Design review of the part shown in the three views and the two pictorial views. Dimensions are in mm from the part's minimum x, y and z. Give positions to 0.01 mm unless a question says otherwise; leave off trailing zeros. Write each loop counter-clockwise with the first axis right and the second up, starting at its lowest first coordinate (ties: lowest second). Pieces come first, ordered by that corner, then holes. Notation, with made-up numbers: M 14,18 L 56,18 A10 cw 56,34 Z; hole C 4.5,-7.75 d7. An arc over 180 degrees is marked long. Use one line per item in the form item = value. Start each with the question number.
Q1. Consider section D-D on z = 14. Write out the cut boundary in (x, y) (3 decimals).
Q2. For probe 1 along X at (y, z) = (2.5, 16.05) (3 decimals); probe 2 along Y at (x, z) = (1.1, 15.5) (1 decimal); probe 3 along Y at (x, z) = (1.05, 2.5) (1 decimal), list the stretches that pass through material, from the lowest coordinate up. Write a range as [from, to].
Q3. Clearance check with flat-ended pins moving along their axes: pin 1 Ø2 at (x, z) = (3.5, 3.5) entering from -Y; pin 2 Ø1 at (x, z) = (2.5, 12) entering from -Y; pin 3 Ø2 at (x, y) = (2.17, 2.5) entering from +Z. State where each tip first meets the part, or that it passes through.
Q4. Consider section C-C on x = 0.4. Write out the cut boundary in (y, z), and give its area (3 significant figures).
Q5. Mouldability with a two-part tool opening along Y and no side actions: class the marked faces 1, 2, 3 and 4 as released by +Y, released by -Y, zero draft, split by the parting line, or undercut.
Q6. Consider section A-A on z = 2.75. Write out the cut boundary in (x, y) (3 decimals).
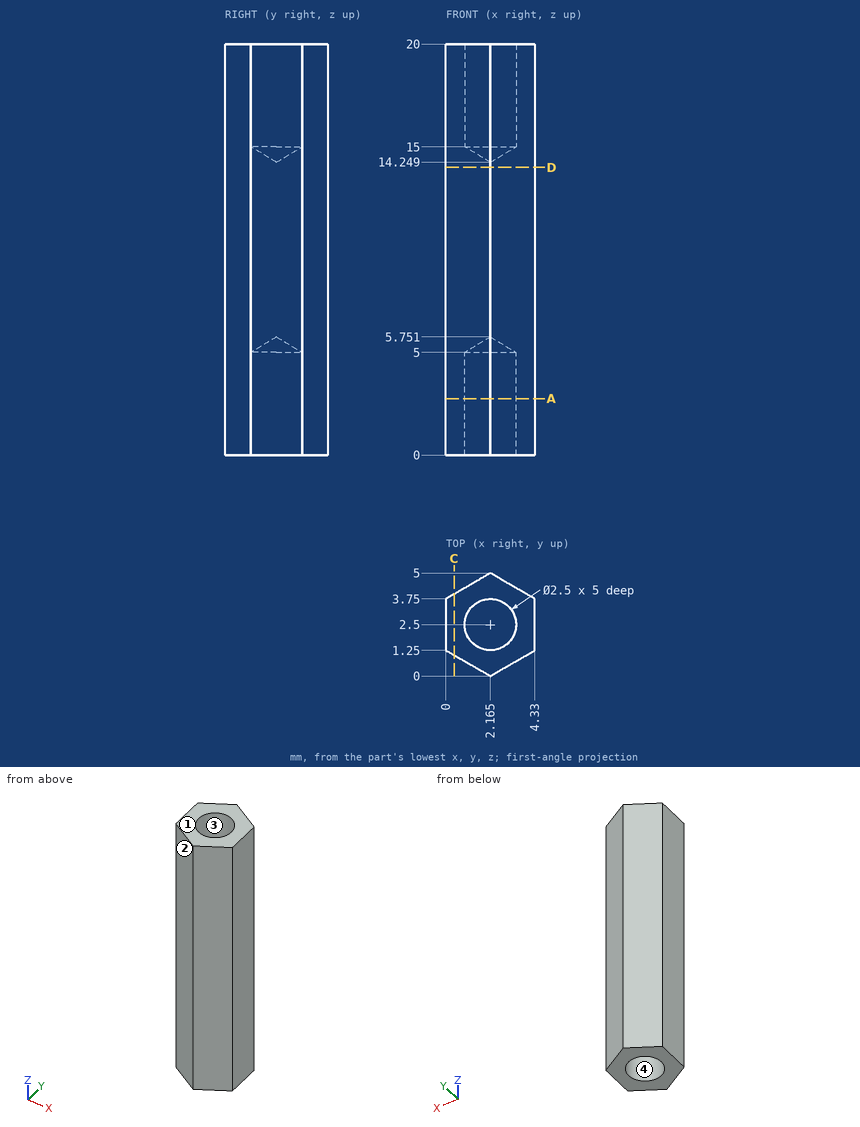
Working result:
q1.outline = M 0,1.25 L 2.165,0 L 4.33,1.25 L 4.33,3.75 L 2.165,5 L 0,3.75 Z
q2.probe_1 = [0, 0.915], [3.415, 4.33]
q2.probe_2 = [0.6, 1.8], [3.2, 4.4]
q2.probe_3 = [0.6, 1.9], [3.1, 4.4]
q3.pin_1 = 0.19
q3.pin_2 = 0
q3.pin_3 = 14.85
q4.outline = M 1.02,0 L 3.98,0 L 3.98,20 L 1.02,20 Z
q4.area = 59.2 mm²
q5.face_1 = zero draft
q5.face_2 = released by -Y
q5.face_3 = undercut
q5.face_4 = undercut
q6.outline = M 0,1.25 L 2.165,0 L 4.33,1.25 L 4.33,3.75 L 2.165,5 L 0,3.75 Z; hole C 2.165,2.5 d2.5
